```python
from build123d import *

# Parameters (mm, degrees)
AUFSATZ_LINEAR_AUSTRAGEN1_DEPTH = 1
VERRUNDUNG1_R                   = 0.5
SKIZZE2_R                       = 1.75
SKIZZE2_R_2                     = 0.75
AUFSATZ_LINEAR_AUSTRAGEN2_DEPTH = 5


with BuildPart() as part:
    # Skizze1 → Aufsatz-Linear austragen1 (new body)
    with BuildSketch(Plane.XY):
        with BuildLine():
            Line((-3.25, 9), (-3.25, 2))
            Line((-3.25, 2), (-1.75, -2))
            Line((-1.75, -2), (1.75, -2))
            Line((1.75, -2), (3.25, 2))
            Line((3.25, 2), (3.25, 9))
            Line((3.25, 9), (2.25, 9))
            Line((2.25, 9), (2.25, 4.25))
            ThreePointArc((2.25, 4.25), (0, 2), (-2.25, 4.25))
            Line((-2.25, 4.25), (-2.25, 9))
            Line((-2.25, 9), (-3.25, 9))
        make_face()
    extrude(amount=AUFSATZ_LINEAR_AUSTRAGEN1_DEPTH)

    # Verrundung1
    verrundung1_edges = [part.edges().sort_by_distance(p)[0] for p in [
        (-3.25, 2, 0.5),
        (3.25, 2, 0.5),
        (3.25, 9, 0.5),
        (2.25, 9, 0.5),
        (-2.25, 9, 0.5),
        (-3.25, 9, 0.5),
    ]]
    fillet(verrundung1_edges, radius=VERRUNDUNG1_R - 0.0001)  # a hair under: the kernel refuses the full size

    # Skizze2 → Aufsatz-Linear austragen2 (add)
    with BuildSketch(Plane.XZ.offset(2)):
        with Locations(Location((0, 1.75, 0), (0, 0, 205.376933525))):
            Circle(SKIZZE2_R)
        with Locations(Location((0, 1.75, 0), (0, 0, 270))):
            Circle(SKIZZE2_R_2, mode=Mode.SUBTRACT)
    extrude(amount=AUFSATZ_LINEAR_AUSTRAGEN2_DEPTH)


solid = part.part
```
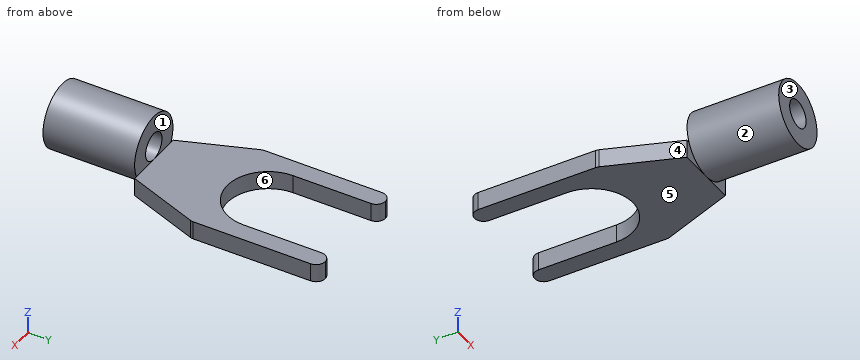
Here's how the part is built. I have some questions about the finished solid (model axes, mm). Face numbers are marked on the shaded views. A direction names the side the tool comes from. Give positions to 0.01 mm unless a question says otherwise; leave off trailing zeros. Write each loop counter-clockwise with the first axis right and the second up, starting at its lowest first coordinate (ties: lowest second). Pieces come first, ordered by that corner, then holes. Notation, with made-up numbers: M 27.25,-4.75 L 49.25,-4.75 A18 cw 49.25,21.25 Z; hole C 84.25,18.25 d10. An arc over 180 degrees is marked long. Put each result on its own line as item: value. Start each with the question number.
Item 1: Will this pin go through, and if not, where does the flat tip stop? pin 1 (1.4 mm diameter, centred on x = 0, z = 1.75, fed in from +Y).
Item 2: I need wall thicknesses on L1, parallel to X at y = -4.05, z = 1.75; L2, parallel to Y at x = 1.5, z = 2.4; L3, parallel to Z at x = -1, y = 2. Which ranges of each line are inside material? Lowest first, please. Write a range as from..to.
Item 3: If we section it at B-B, the plane z = 1.75: Write out the boundary of the cut face in (x, y).
Item 4: If we section it at C-C, the plane z = 3.15: Write out the boundary of the cut face in (x, y), then the cut area to 3 significant figures.
Item 5: Thinking about a two-plate mould opening in X: for the marked faces 4, 5 and 6, which applies, +X half, -X half, draft (parallel to the pull), parting line (faces both ways), or undercut?
Item 6: If we section it at D-D, the plane y = -5.5: Write out the boundary of the cut face in (x, z).
Item 7: If we section it at A-A, the plane y = 5.5: Write out the boundary of the cut face in (x, z).
Item 8: On a 3-axis mill with a long thin cutter (end or side, diameter ignored), from which of +Z, -Z, +X, -X, +Y, -Y can I reach the whole of each face in a straight line? I mean the marked faces 1, 2 and 3. Say none if no direction works.
Values:
1. pin 1: through
2. L1: -1.75..-0.75, 0.75..1.75
2. L2: -7..-2
2. L3: 0..1
3. outline: M -1.75,-7 L -0.75,-7 L -0.75,-2 L -1.75,-2 Z; M 0.75,-7 L 1.75,-7 L 1.75,-2 L 0.75,-2 Z
4. outline: M -1.05,-7 L 1.05,-7 L 1.05,-2 L -1.05,-2 Z
4. area: 10.5 mm²
5. face 4: -X half
5. face 5: draft
5. face 6: undercut
6. outline: C 0,1.75 d3.5; hole C 0,1.75 d1.5
7. outline: M -3.25,0 L -2.25,0 L -2.25,1 L -3.25,1 Z; M 2.25,0 L 3.25,0 L 3.25,1 L 2.25,1 Z
8. face 1: +Z, +X, -X, +Y
8. face 2: -Y
8. face 3: +Z, -Z, +X, -X, -Y
